Source: CAD feature listing. Evaluate the final solid. Frame: model axes, mm. A direction names the side the tool comes from. Give positions to 0.01 mm unless a question says otherwise; leave off trailing zeros. Write each loop counter-clockwise with the first axis right and the second up, starting at its lowest first coordinate (ties: lowest second). Pieces come first, ordered by that corner, then holes. Notation, with made-up numbers: (71, -22) - (83, -22) arc R27 cw to (83, 1) - close; hole circle Ø11 at (44, 32). An arc over 180 degrees is marked (long way). One line per question, with ' | ' between items. Start each with the question number.
(1) Pin query (flat end, axial travel): pin 1 (4.5 mm diameter, centred on x = 6.35, y = 45.212, fed in from -Z). Return the tip coordinate at first contact, or that it passes through.
(2) Section C-C, the plane y = 5.08. Return loops of the section in (x, z).
(3) Ray query, line 1 (X direction, y = 5, z = 3.5); line 2 (Y direction, x = 30, z = 4); line 3 (X direction, y = 32, z = 3.25). Return the intervals inside material, ascending. Write a range as [from, to].
(4) Draft query along X for faces 1 (the cylindrical face through (7.19, 23.782, 3.131)), 2 (the flat face through (0, 25, 3)), 3 (the flat face through (80.01, 25, 3)), 4 (the flat face through (46, 48, 6.35)). Return one class per face: +X half, -X half, draft (parallel to the pull), parting line (faces both ways), or undercut.
(5) Access query for faces 5 (the cylindrical face through (0.955, 49.387, 3.131)), 6 (the flat face through (47, 6.731, 3)). Directions: +Z, -Z, +X, -X, +Y, -Y. A direction counts if a zero-diameter tool reaches every point of the face in a straight line with its end or side. Return the directions, or none.
(6) Section D-D, the plane z = 4. Return loops of the section in (x, y) (3 decimals), plus the area to 3 significant figures.
(7) Section B-B, the plane y = 16.5. Return loops of the section in (x, z), plus the area to 3 significant figures.
(8) Section A-A, the plane x = 57. Return loops of the section in (y, z).
```python
from build123d import *

# Parameters (mm, degrees)
F0_R     = 1.397
F1_DEPTH = 6.35


with BuildPart() as f1:
    # F0 (on Top) → F1 (new body)
    with BuildSketch(Plane.XY):
        with BuildLine():
            ThreePointArc((0, 3.175), (0.929936, 0.929936), (3.175, 0))
            Line((3.175, 0), (90.805, 0))
            ThreePointArc((90.805, 0), (93.050064, 0.929936), (93.98, 3.175))
            Line((93.98, 3.175), (93.98, 47.117))
            ThreePointArc((93.98, 47.117), (93.050064, 49.362064), (90.805, 50.292))
            Line((90.805, 50.292), (3.175, 50.292))
            ThreePointArc((3.175, 50.292), (0.929936, 49.362064), (0, 47.117))
            Line((0, 47.117), (0, 3.175))
        make_face()
        with Locations((6.35, 5.08)):
            Circle(F0_R, mode=Mode.SUBTRACT)
        with Locations((7.493, 25.146)):
            Circle(F0_R, mode=Mode.SUBTRACT)
        with BuildLine():
            Line((76.835, 6.731), (17.145, 6.731))
            ThreePointArc((17.145, 6.731), (14.899936, 7.660936), (13.97, 9.906))
            Line((13.97, 9.906), (13.97, 40.386))
            ThreePointArc((13.97, 40.386), (14.899936, 42.631064), (17.145, 43.561))
            Line((17.145, 43.561), (76.835, 43.561))
            ThreePointArc((76.835, 43.561), (79.080064, 42.631064), (80.01, 40.386))
            Line((80.01, 40.386), (80.01, 9.906))
            ThreePointArc((80.01, 9.906), (79.080064, 7.660936), (76.835, 6.731))
        make_face(mode=Mode.SUBTRACT)
        with Locations((87.63, 5.08)):
            Circle(F0_R, mode=Mode.SUBTRACT)
        with Locations((86.487, 25.146)):
            Circle(F0_R, mode=Mode.SUBTRACT)
        with Locations((6.35, 45.212)):
            Circle(F0_R, mode=Mode.SUBTRACT)
        with Locations((87.63, 45.212)):
            Circle(F0_R, mode=Mode.SUBTRACT)
    extrude(amount=F1_DEPTH)


solid = f1.part
```
Check sheet entries:
1) pin 1: z = 0
2) outline: (0, 0) - (4.95, 0) - (4.95, 6.35) - (0, 6.35) - close; (7.75, 0) - (86.23, 0) - (86.23, 6.35) - (7.75, 6.35) - close; (89.03, 0) - (93.98, 0) - (93.98, 6.35) - (89.03, 6.35) - close
3) line 1: [0, 4.96], [7.74, 86.24], [89.02, 93.98] | line 2: [0, 6.73], [43.56, 50.29] | line 3: [0, 13.97], [80.01, 93.98]
4) face 1: undercut | face 2: -X half | face 3: undercut | face 4: draft
5) face 5: +Z, -Z, -X, +Y | face 6: +Z, -Z
6) outline: (0, 3.175) arc R3.175 ccw to (3.175, 0) - (90.805, 0) arc R3.175 ccw to (93.98, 3.175) - (93.98, 47.117) arc R3.175 ccw to (90.805, 50.292) - (3.175, 50.292) arc R3.175 ccw to (0, 47.117) - close; hole circle Ø2.794 at (6.35, 5.08); hole circle Ø2.794 at (6.35, 45.212); hole circle Ø2.794 at (7.493, 25.146); hole (13.97, 9.906) arc R3.175 ccw to (17.145, 6.731) - (76.835, 6.731) arc R3.175 ccw to (80.01, 9.906) - (80.01, 40.386) arc R3.175 ccw to (76.835, 43.561) - (17.145, 43.561) arc R3.175 ccw to (13.97, 40.386) - close; hole circle Ø2.794 at (86.487, 25.146); hole circle Ø2.794 at (87.63, 5.08); hole circle Ø2.794 at (87.63, 45.212) | area: 2,260 mm²
7) outline: (0, 0) - (13.97, 0) - (13.97, 6.35) - (0, 6.35) - close; (80.01, 0) - (93.98, 0) - (93.98, 6.35) - (80.01, 6.35) - close | area: 177 mm²
8) outline: (0, 0) - (6.73, 0) - (6.73, 6.35) - (0, 6.35) - close; (43.56, 0) - (50.29, 0) - (50.29, 6.35) - (43.56, 6.35) - close
